from build123d import *

# Parameters (mm, degrees)
SKETCH1_W           = 43.1509
SKETCH1_H           = 60.58823
BOSS_EXTRUDE1_DEPTH = 2
FILLET1_R           = 4
SKETCH2_R           = 1.0922
CUT_EXTRUDE1_DEPTH  = 2
BOSS_EXTRUDE2_DEPTH = 3.333333333
CUT_EXTRUDE2_REACH  = 48.51
SKETCH6_R           = 3


with BuildPart() as part:
    # Sketch1 → Boss-Extrude1 (new body)
    with BuildSketch(Plane.XY):
        Rectangle(SKETCH1_W, SKETCH1_H)
    extrude(amount=BOSS_EXTRUDE1_DEPTH)

    # Fillet1
    fillet1_edges = [part.edges().sort_by_distance(p)[0] for p in [
        (21.57545, -30.294115, 1),
        (-21.57545, -30.294115, 1),
        (-21.57545, 30.294115, 1),
        (21.57545, 30.294115, 1),
    ]]
    fillet(fillet1_edges, radius=FILLET1_R)

    # Sketch2 → Cut-Extrude1 (cut)
    with BuildSketch(Plane.XY.offset(2)):
        with Locations((-16.57545, 25.294115)):
            Circle(SKETCH2_R)
        with Locations((16.57545, 25.294115)):
            Circle(SKETCH2_R)
        with Locations((-16.57545, -25.294115)):
            Circle(SKETCH2_R)
        with Locations((16.57545, -25.294115)):
            Circle(SKETCH2_R)
    extrude(amount=-CUT_EXTRUDE1_DEPTH, mode=Mode.SUBTRACT)

    # Sketch5 → Boss-Extrude2 (add, symmetric)
    with BuildSketch(Plane(origin=(0, 0, 0), x_dir=(0, 0, -1), z_dir=(1, 0, 0))):
        with BuildLine():
            Line((0, 25), (0, -25))
            ThreePointArc((0, -25), (25, 0), (0, 25))
        make_face()
    extrude(amount=BOSS_EXTRUDE2_DEPTH, both=True)

    # Sketch6 → Cut-Extrude2 (cut, up to next)
    with BuildSketch(Plane(origin=(3.333333333, 0, 0), x_dir=(0, 0, -1), z_dir=(1, 0, 0)), mode=Mode.PRIVATE) as cut_extrude2_sk1:
        with Locations((10.61, 0)):
            Circle(SKETCH6_R)
    cut_extrude2_tool1 = extrude(cut_extrude2_sk1.sketch, amount=-CUT_EXTRUDE2_REACH, mode=Mode.PRIVATE) & part.part
    add(cut_extrude2_tool1.solids().sort_by_distance((3.333333, 0, -10.61))[0], mode=Mode.SUBTRACT)


solid = part.part
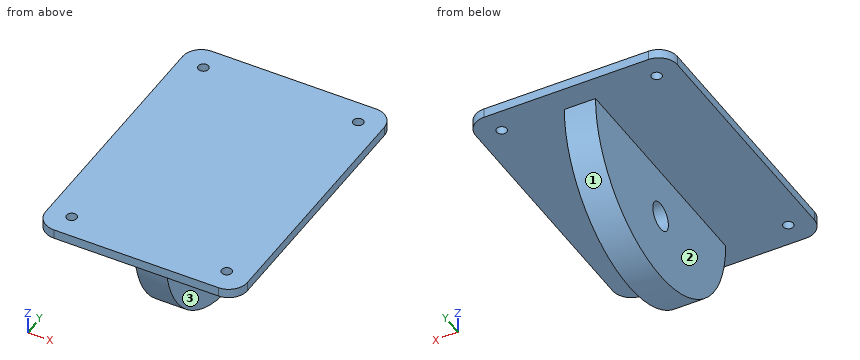
Work out the finished part from the listing and answer in its coordinate system (mm). Face numbers are marked on the shaded views. A direction names the side the tool comes from. Give positions to 0.01 mm unless a question says otherwise; leave off trailing zeros. Loops run counter-clockwise (first coordinate to the right, second up) from the corner with the lowest first, then second, coordinate; pieces in that order, holes last. Notation, with made-up numbers: (21.25, 87.5) - (58.25, 87.5) arc R28 cw to (58.25, 119.5) - close; hole circle Ø11 at (5, 16). An arc over 180 degrees is marked (long way). Answer in a Markdown table with one row per item. Add a question column.
Q1. Each of these flat-tipped pins is pushed along its axis until it touches: P1, Ø1.5, axis at y = -10.5, z = -8.5, coming from the +X side; P2, Ø6, axis at x = 2.5, z = -19.5, coming from the -Y side; P3, Ø5, axis at y = -22, z = -8.5, coming from the -X side. Where does it stop, or does it pass through?
Q2. Consider line 1 along X through (y, z) = (-2, -14); line 2 along Z through (x, y) = (17.5, -15); line 3 along Y through (x, z) = (-0.25, -10.61). Determine where each line is inside the solid, lowest interval first.
Q3. The part is cut by section A-A (y = 0). Determine the outline of the cut face in (x, z).
Q4. The part is cut by section B-B (x = 1). Determine the outline of the cut face in (y, z).
Q5. A tool of negligible diameter and unlimited length cuts with its end or side. For the marked faces 1, 2 and 3, from which of +Z, -Z, +X, -X, +Y, -Y can it reach the whole face along a straight path? Write none if from no direction.
Q6. The part is cut by section C-C (z = -11.5). Determine the outline of the cut face in (x, y), and give its area (3 significant figures).
Q7. The part is cut by section D-D (y = 18.5). Determine the outline of the cut face in (x, z), and give its area (3 significant figures).
Solution:
| question | item | result |
|---|---|---|
| 1 | P1 | stops at x = 3.33 |
| 1 | P2 | stops at y = -18.78 |
| 1 | P3 | stops at x = -3.33 |
| 2 | line 1 | x = -3.33 to 3.33 |
| 2 | line 2 | z = 0 to 2 |
| 2 | line 3 | y = -22.64 to -3, 3 to 22.64 |
| 3 | outline | (-21.58, 0) - (-3.33, 0) - (-3.33, -7.61) - (3.33, -7.61) - (3.33, 0) - (21.58, 0) - (21.58, 2) - (-21.58, 2) - close; (-3.33, -25) - (3.33, -25) - (3.33, -13.61) - (-3.33, -13.61) - close |
| 4 | outline | (-30.29, 0) - (-25, 0) arc R25 ccw to (25, 0) - (30.29, 0) - (30.29, 2) - (-30.29, 2) - close; hole circle Ø6 at (0, -10.61) |
| 5 | face 1 | -Z, +X, -X |
| 5 | face 2 | -Z, -X, +Y, -Y |
| 5 | face 3 | -Z, +X, +Y, -Y |
| 6 | outline | (-3.33, -22.2) - (3.33, -22.2) - (3.33, -2.86) - (-3.33, -2.86) - close; (-3.33, 2.86) - (3.33, 2.86) - (3.33, 22.2) - (-3.33, 22.2) - close |
| 6 | area | 258 mm² |
| 7 | outline | (-21.58, 0) - (-3.33, 0) - (-3.33, -16.82) - (3.33, -16.82) - (3.33, 0) - (21.58, 0) - (21.58, 2) - (-21.58, 2) - close |
| 7 | area | 198 mm² |
